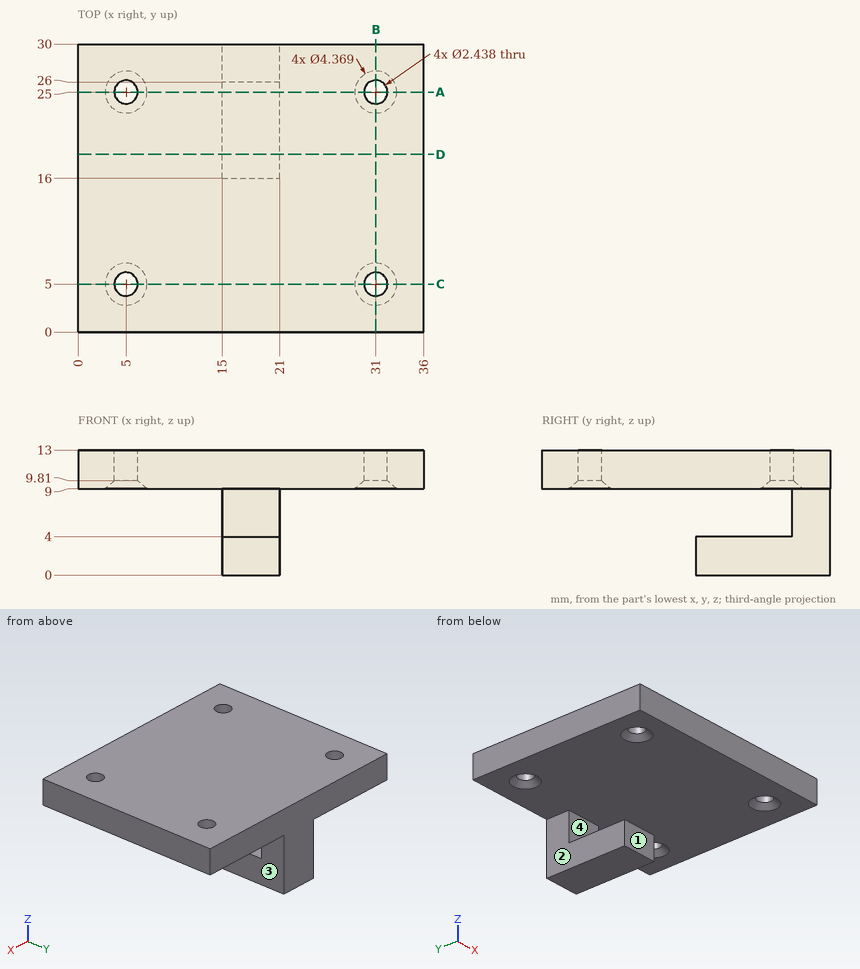
Geometry check sheet. Reference: drawing and pictorial views, mm from the part's lowest x, y, z. A direction names the side the tool comes from. Give positions to 0.01 mm unless a question says otherwise; leave off trailing zeros. Write each loop counter-clockwise with the first axis right and the second up, starting at its lowest first coordinate (ties: lowest second). Pieces come first, ordered by that corner, then holes. Notation, with made-up numbers: (-31.5, 42.5) -> (1.5, 42.5) arc R26 cw to (1.5, 57.5) -> close; hole circle Ø11 at (60, -38). An arc over 180 degrees is marked (long way). One line per question, with ' | ' between items.
Item 1: Access from +Z, -Z, +X, -X, +Y, -Y to the whole of each face (thin tool, end or side, straight path). Record for the marked faces 1, 2, 3 and 4.
Determined:
face 1: -Z, +X, -X, -Y | face 2: -Z, -X, +Y, -Y | face 3: -Z, +X, +Y, -Y | face 4: +X, -X, -Y
Item 2: Depth check by flat-ended pin: pin 1 (3 mm diameter, centred on x = 21.5, y = 5.5, fed in from -Z); pin 2 (2.5 mm diameter, centred on y = 21, z = 3, fed in from -X); pin 3 (7 mm diameter, centred on y = 20, z = 2.5, fed in from +X); pin 4 (1.5 mm diameter, centred on x = 31, y = 25, fed in from +Z). Enter the tip coordinate at first touch or a pass-through.
Determined:
pin 1: z = 9 | pin 2: x = 15 | pin 3: x = 21 | pin 4: through
Item 3: Scan lines: line 1 along X through (y, z) = (25, 10.6); line 2 along Y through (x, z) = (31, 12.05); line 3 along Z through (x, y) = (20, 14.5). Record each from-to range of solid material in increasing order.
Determined:
line 1: 0 to 3.78, 6.22 to 29.78, 32.22 to 36 | line 2: 0 to 3.78, 6.22 to 23.78, 26.22 to 30 | line 3: 9 to 13
Item 4: Sectioned sample at D-D, the plane y = 18.5. Record the boundary of the cut face in (x, z), plus the area to 3 significant figures.
Determined:
outline: (0, 9) -> (36, 9) -> (36, 13) -> (0, 13) -> close; (15, 0) -> (21, 0) -> (21, 4) -> (15, 4) -> close | area: 168 mm^2
Item 5: Sectioned sample at A-A, the plane y = 25. Record the boundary of the cut face in (x, z) (1 decimal), plus the area to 3 significant figures.
Determined:
outline: (0, 9) -> (2.8, 9) -> (3.8, 9.8) -> (3.8, 13) -> (0, 13) -> close; (6.2, 9.8) -> (7.2, 9) -> (28.8, 9) -> (29.8, 9.8) -> (29.8, 13) -> (6.2, 13) -> close; (15, 0) -> (21, 0) -> (21, 4) -> (15, 4) -> close; (32.2, 9.8) -> (33.2, 9) -> (36, 9) -> (36, 13) -> (32.2, 13) -> close | area: 147 mm^2
Item 6: Sectioned sample at C-C, the plane y = 5. Record the boundary of the cut face in (x, z) (1 decimal), plus the area to 3 significant figures.
Determined:
outline: (0, 9) -> (2.8, 9) -> (3.8, 9.8) -> (3.8, 13) -> (0, 13) -> close; (6.2, 9.8) -> (7.2, 9) -> (28.8, 9) -> (29.8, 9.8) -> (29.8, 13) -> (6.2, 13) -> close; (32.2, 9.8) -> (33.2, 9) -> (36, 9) -> (36, 13) -> (32.2, 13) -> close | area: 123 mm^2
Item 7: Sectioned sample at B-B, the plane x = 31. Record the boundary of the cut face in (y, z) (1 decimal).
Determined:
outline: (0, 9) -> (2.8, 9) -> (3.8, 9.8) -> (3.8, 13) -> (0, 13) -> close; (6.2, 9.8) -> (7.2, 9) -> (22.8, 9) -> (23.8, 9.8) -> (23.8, 13) -> (6.2, 13) -> close; (26.2, 9.8) -> (27.2, 9) -> (30, 9) -> (30, 13) -> (26.2, 13) -> close
